CAD build for the part. Positions are in the model's coordinates, mm. A direction names the side the tool comes from. Coordinates: 2 decimals unless noted, no trailing zeros. Loops run counter-clockwise (first coordinate to the right, second up) from the corner with the lowest first, then second, coordinate; pieces in that order, holes last.
1) Wall check: line 1 along Y through (x, z) = (0, 2.9); line 2 along Y through (x, z) = (2, 2.25); line 3 along Y through (x, z) = (-23, 1.75). Give the ranges that are in metal, low to high.
2) Saw through at B-B, the plane x = 0. Give the number of separate pieces and of enclosed holes in the cut face, and give its area (3 significant figures).
3) Two-plate mould, pull along X, no slides. Class faces 4 (the flat face through (-21, -11, 6)), 5 (the flat face through (1.5, 9, 4)), 6 (the cylindrical face through (0, -22, 4)): +X half, -X half, draft (parallel to the pull), parting line (faces both ways), or undercut.
4) Pin check, flat tips, straight feed: pin 1 Ø3 at (x, y) = (14, -16.5) entering from -Z; pin 2 Ø1 at (x, y) = (-20, -15) entering from +Z; pin 3 Ø2.5 at (x, y) = (-23, 0) entering from -Z. Stop position of each tip, or through.
5) Saw through at C-C, the plane x = 8. Write the cut outline in (y, z), and give its area (3 significant figures).
6) Which spindle directions (+Z, -Z, +X, -X, +Y, -Y) get a long thin tool onto all of the face, cutting with end or side? Do faces 1 (the flat face through (20.5, 5, 4)), 2 (the flat face through (-10.5, 18, 5)), 3 (the cylindrical face through (2.93, -21.1, 4.03)). Say none if no direction does.
7) Saw through at A-A, the plane z = 7. Write the cut outline in (x, y), and give its area (3 significant figures).
```python
from build123d import *

# Parameters (mm, degrees)
F1_DEPTH         = 2
F2_W             = 5
F2_H             = 5
F3_DEPTH         = 4
F4_DEPTH         = 6
F5_R             = 1
F7_D             = 2
F7_CBORE_D       = 4.2
F7_CBORE_DEPTH   = 1.5
F2_W_2           = 15
F2_H_2           = 13
F8_DEPTH         = 25
F9_SIZE          = 1.99999
F10_R            = 1.5
F11_DEPTH        = 4
F14_DEPTH        = 6
F16_DEPTH        = 1.5
F18_DEPTH        = 1
F19_D            = 3
F20_W            = 4
F20_H            = 4
F21_DEPTH        = 4
F22_R            = 0.99999
F24_D            = 1.8
F24_DEPTH        = 5
F24_TIP          = 0.5407745571
F24_ON_F13_D     = 1.8
F24_ON_F13_DEPTH = 5
F24_ON_F13_TIP   = 0.5407745571
F24_ON_F23_D     = 1.8
F24_ON_F23_DEPTH = 5
F24_ON_F23_TIP   = 0.5407745571
F25_DEPTH        = 3
F27_DEPTH        = 2.5
F28_SIZE         = 1.99999
F29_R            = 0.99999
F30_DEPTH        = 1
F31_DEPTH        = 1
F32_DEPTH        = 1
F33_DEPTH        = 1
F34_R            = 2
F36_D            = 1.8
F36_DEPTH        = 5
F36_TIP          = 0.5407745571


# Not quite as in the source:
# - a fillet or chamfer is up to 0.001 mm smaller than in the source, because OpenCascade refuses the exact size
# - a feature names something its author has since deleted; it is built from what else it names


with BuildPart() as f1:
    # F0 (on Top) → F1 (new body)
    with BuildSketch(Plane.XY):
        with BuildLine():
            Line((-24.5, -25.5), (24.5, -25.5))
            ThreePointArc((24.5, -25.5), (25.2071067812, -25.2071067812), (25.5, -24.5))
            Line((25.5, -24.5), (25.5, 24.5))
            ThreePointArc((25.5, 24.5), (25.2071067812, 25.2071067812), (24.5, 25.5))
            Line((24.5, 25.5), (-24.5, 25.5))
            ThreePointArc((-24.5, 25.5), (-25.2071067812, 25.2071067812), (-25.5, 24.5))
            Line((-25.5, 24.5), (-25.5, -24.5))
            ThreePointArc((-25.5, -24.5), (-25.2071067812, -25.2071067812), (-24.5, -25.5))
        make_face()
    extrude(amount=F1_DEPTH)

    # F2 (on face) → F3 (join)
    with BuildSketch(Plane.XY.offset(2)):
        with Locations((-23, 0)):
            Rectangle(F2_W, F2_H)
        with Locations((0, 23)):
            Rectangle(F2_W, F2_H)
        with Locations((23, 5)):
            Rectangle(F2_W, F2_H)
        with Locations((0, -23)):
            Rectangle(F2_W, F2_H)
    extrude(amount=F3_DEPTH)

    # F2 (on face) → F4 (join)
    with BuildSketch(Plane.XY.offset(2)):
        with BuildLine():
            Line((-25.5, 24.5), (-25.5, 10.5))
            Line((-25.5, 10.5), (-10.5, 10.5))
            Line((-10.5, 10.5), (-10.5, 25.5))
            Line((-10.5, 25.5), (-24.5, 25.5))
            ThreePointArc((-24.5, 25.5), (-25.2071067812, 25.2071067812), (-25.5, 24.5))
        make_face()
    extrude(amount=F4_DEPTH)

    # F5
    f5_edges = [f1.edges().sort_by_distance(p)[0] for p in [
        (-10.5, 10.5, 5),
    ]]
    fillet(f5_edges, radius=F5_R)

    # F7 (through all)
    with Locations(Plane(origin=(0, 0, 0), x_dir=(1, 0, 0), z_dir=(0, 0, -1))):
        with Locations((-23, 0), (0, 23), (23, -5), (0, -23)):
            CounterBoreHole(F7_D / 2, F7_CBORE_D / 2, F7_CBORE_DEPTH)

    # F2 (on face) → F8 (cut)
    with BuildSketch(Plane.XY.offset(2)):
        with Locations((-3.5, -8.5)):
            Rectangle(F2_W_2, F2_H_2)
    extrude(amount=-F8_DEPTH, mode=Mode.SUBTRACT)

    # F9 (size 2 in the source; OpenCascade refuses exactly that, so slightly less here)
    f9_edges = [f1.edges().sort_by_distance(p)[0] for p in [
        (-11, -8.5, 0),
        (-3.5, -15, 0),
        (4, -8.5, 0),
        (-3.5, -2, 0),
    ]]
    chamfer(f9_edges, length=F9_SIZE)

    # F10 (on face) → F11 (join)
    with BuildSketch(Plane.XY.offset(2)):
        with BuildLine():
            Line((-24.5, -25.5), (-16.5, -25.5))
            Line((-16.5, -25.5), (-16.5, -6.5))
            Line((-16.5, -6.5), (-17.5, -5.5))
            Line((-17.5, -5.5), (-17.5, -3.5))
            ThreePointArc((-17.5, -3.5), (-17.7928932188, -2.7928932188), (-18.5, -2.5))
            Line((-18.5, -2.5), (-20.5, -2.5))
            Line((-20.5, -2.5), (-25.5, -2.5))
            Line((-25.5, -2.5), (-25.5, -24.5))
            ThreePointArc((-25.5, -24.5), (-25.2071067812, -25.2071067812), (-24.5, -25.5))
        make_face()
        with Locations((-14, -4)):
            Circle(F10_R)
    extrude(amount=F11_DEPTH)

    # F13 (on face) → F14 (cut)
    with BuildSketch(Plane.XY.offset(8)):
        Polygon((-14.5, 12.5), (-12.5, 12.5), (-12.5, 20.5), (-23.5, 20.5), (-23.5, 12.5), (-18.5, 12.5), (-18.5, 10.5), (-14.5, 10.5), align=None)
    extrude(amount=-F14_DEPTH, mode=Mode.SUBTRACT)

    # F15 (on face) → F16 (cut)
    with BuildSketch(Plane(origin=(0, 0, 0), x_dir=(1, 0, 0), z_dir=(0, 0, -1))):
        with BuildLine():
            ThreePointArc((-2.1, 23), (0, 25.1), (2.1, 23))
            Line((2.1, 23), (2.1, 25.5))
            Line((2.1, 25.5), (-2.1, 25.5))
            Line((-2.1, 25.5), (-2.1, 23))
        make_face()
        with BuildLine():
            Line((25.5, -7.1), (25.5, -2.9))
            Line((25.5, -2.9), (23, -2.9))
            ThreePointArc((23, -2.9), (24.4849242405, -3.5150757595), (25.1, -5))
            ThreePointArc((25.1, -5), (24.4849242405, -6.4849242405), (23, -7.1))
            Line((23, -7.1), (25.5, -7.1))
        make_face()
        with BuildLine():
            Line((-23, 2.1), (-25.5, 2.1))
            Line((-25.5, 2.1), (-25.5, -2.1))
            Line((-25.5, -2.1), (-23, -2.1))
            ThreePointArc((-23, -2.1), (-25.1, 0), (-23, 2.1))
        make_face()
        with BuildLine():
            Line((-2.1, -25.5), (2.1, -25.5))
            Line((2.1, -25.5), (2.1, -23))
            ThreePointArc((2.1, -23), (0, -25.1), (-2.1, -23))
            Line((-2.1, -23), (-2.1, -25.5))
        make_face()
    extrude(amount=-F16_DEPTH, mode=Mode.SUBTRACT)

    # F17 (on face) → F18 (cut)
    with BuildSketch(Plane(origin=(0, 0, 0), x_dir=(1, 0, 0), z_dir=(0, 0, -1))):
        Polygon((17.25, 18.0877132403), (14.5, 19.6754264805), (11.75, 18.0877132403), (11.75, 14.9122867597), (14.5, 13.3245735195), (17.25, 14.9122867597), align=None)
        Polygon((17.25, -0.0877132403), (17.25, 3.0877132403), (14.5, 4.6754264805), (11.75, 3.0877132403), (11.75, -0.0877132403), (14.5, -1.6754264805), align=None)
    extrude(amount=-F18_DEPTH, mode=Mode.SUBTRACT)

    # F19 (through all)
    with Locations(Plane(origin=(0, 0, 0), x_dir=(1, 0, 0), z_dir=(0, 0, -1))):
        with Locations((14.5, 16.5), (14.5, 1.5)):
            Hole(F19_D / 2)

    # F20 (on face) → F21 (join)
    with BuildSketch(Plane.XY.offset(2)):
        with Locations((23.5, 9.5)):
            Rectangle(F20_W, F20_H)
        with Locations((3.5, 9.5)):
            Rectangle(F20_W, F20_H)
        with BuildLine():
            Line((2.5, 20.5), (25.5, 20.5))
            Line((25.5, 20.5), (25.5, 24.5))
            ThreePointArc((25.5, 24.5), (25.2071067812, 25.2071067812), (24.5, 25.5))
            Line((24.5, 25.5), (2.5, 25.5))
            Line((2.5, 25.5), (2.5, 20.5))
        make_face()
        with BuildLine():
            Line((25.5, -24.5), (25.5, -20.5))
            Line((25.5, -20.5), (20.5, -20.5))
            Line((20.5, -20.5), (20.5, -25.5))
            Line((20.5, -25.5), (24.5, -25.5))
            ThreePointArc((24.5, -25.5), (25.2071067812, -25.2071067812), (25.5, -24.5))
        make_face()
    extrude(amount=F21_DEPTH)

    # F22 (radius 1 in the source; OpenCascade refuses exactly that, so slightly less here)
    f22_edges = [f1.edges().sort_by_distance(p)[0] for p in [
        (5.5, 7.5, 4),
        (1.5, 7.5, 4),
        (1.5, 11.5, 4),
        (20.5, 7.5, 4),
        (5.5, 11.5, 4),
        (21.5, 11.5, 4),
    ]]
    fillet(f22_edges, radius=F22_R)

    # F24
    with Locations(Plane.XY.offset(6)):
        with Locations((-22, -22), (-22, -7)):
            Hole(F24_D / 2, depth=F24_DEPTH)
            with Locations((0, 0, -(F24_DEPTH + F24_TIP / 2))):  # 118° drill point
                Cone(0, F24_D / 2, F24_TIP, mode=Mode.SUBTRACT)

    # F24 on F13
    with Locations(Plane.XY.offset(8)):
        with Locations((-22.5, 22.5), (-13.5, 22.5)):
            Hole(F24_ON_F13_D / 2, depth=F24_ON_F13_DEPTH)
            with Locations((0, 0, -(F24_ON_F13_DEPTH + F24_ON_F13_TIP / 2))):  # 118° drill point
                Cone(0, F24_ON_F13_D / 2, F24_ON_F13_TIP, mode=Mode.SUBTRACT)

    # F24 on F23
    with Locations(Plane.XY.offset(6)):
        with Locations((3.5, 9.5), (23.5, 9.5)):
            Hole(F24_ON_F23_D / 2, depth=F24_ON_F23_DEPTH)
            with Locations((0, 0, -(F24_ON_F23_DEPTH + F24_ON_F23_TIP / 2))):  # 118° drill point
                Cone(0, F24_ON_F23_D / 2, F24_ON_F23_TIP, mode=Mode.SUBTRACT)

    # F25 (add): a face of the model
    f25_faces = [f1.faces().sort_by_distance(p)[0] for p in [
        (-23.5, 16.5, 5),
    ]]
    extrude(f25_faces, amount=F25_DEPTH)

    # F26 (on face) → F27 (cut)
    with BuildSketch(Plane(origin=(0, 0, 0), x_dir=(1, 0, 0), z_dir=(0, 0, -1))):
        with BuildLine():
            Line((-20.5, -21.5), (-21.5, -21.5))
            Line((-21.5, -21.5), (-25.5, -21.5))
            Line((-25.5, -21.5), (-25.5, -24.5))
            ThreePointArc((-25.5, -24.5), (-25.2071067812, -25.2071067812), (-24.5, -25.5))
            Line((-24.5, -25.5), (-21.5, -25.5))
            Line((-21.5, -25.5), (-21.5, -24.5))
            Line((-21.5, -24.5), (-15, -24.5))
            Line((-15, -24.5), (-15, -21))
            Line((-15, -21), (-15, -18.5))
            Line((-15, -18.5), (-20.5, -18.5))
            Line((-20.5, -18.5), (-20.5, -21.5))
        make_face()
    extrude(amount=-F27_DEPTH, mode=Mode.SUBTRACT)

    # F28 (size 2 in the source; OpenCascade refuses exactly that, so slightly less here)
    f28_edges = [f1.edges().sort_by_distance(p)[0] for p in [
        (-17.75, 18.5, 2),
    ]]
    chamfer(f28_edges, length=F28_SIZE)

    # F29 (radius 1 in the source; OpenCascade refuses exactly that, so slightly less here)
    f29_edges = [f1.edges().sort_by_distance(p)[0] for p in [
        (-25.5, 21.5, 1.25),
        (-21.5, 24.5, 1.25),
        (-15, 24.5, 1.25),
    ]]
    fillet(f29_edges, radius=F29_R)

    # F30 (add): faces of the model
    f30_faces = [f1.faces().sort_by_distance(p)[0] for p in [
        (-2.5, 23, 4),
        (-2.5, -23, 4),
        (20.5, -23, 4),
    ]]
    extrude(f30_faces, amount=F30_DEPTH)

    # F31 (add): a face of the model
    f31_faces = [f1.faces().sort_by_distance(p)[0] for p in [
        (2.5, -23, 4),
    ]]
    extrude(f31_faces, amount=F31_DEPTH)

    # F32 (add): a face of the model
    f32_faces = [f1.faces().sort_by_distance(p)[0] for p in [
        (23, 2.5, 4),
    ]]
    extrude(f32_faces, amount=F32_DEPTH)

    # F33 (add): a face of the model
    f33_faces = [f1.faces().sort_by_distance(p)[0] for p in [
        (-23, 2.5, 4),
    ]]
    extrude(f33_faces, amount=F33_DEPTH)

    # F34
    f34_edges = [f1.edges().sort_by_distance(p)[0] for p in [
        (19.5, -20.5, 4),
        (20.5, 1.5, 4),
        (3.5, -20.5, 4),
        (-3.5, -20.5, 4),
        (-3.5, 20.5, 4),
        (-20.5, 3.5, 4),
    ]]
    fillet(f34_edges, radius=F34_R)

    # F36
    with Locations(Plane(origin=(0, 0, 0), x_dir=(1, 0, 0), z_dir=(0, 0, -1))):
        with Locations((-23, -18.5), (-23, 18.5), (23, -23), (23, 23)):
            Hole(F36_D / 2, depth=F36_DEPTH)
            with Locations((0, 0, -(F36_DEPTH + F36_TIP / 2))):  # 118° drill point
                Cone(0, F36_D / 2, F36_TIP, mode=Mode.SUBTRACT)


solid = f1.part
```
Data:
1. line 1: y = -25.5 to -24, -22 to -20.5, 20.5 to 22, 24 to 25.5
1. line 2: y = -25.5 to -20.56, 7.63 to 11.37, 20.5 to 25.5
1. line 3: y = -25.5 to -19.4, -17.6 to -1, 1 to 17.6, 19.4 to 21.5
2. separate pieces: 4
2. enclosed holes: 0
2. area: 80.2 mm2
3. face 4: draft
3. face 5: -X half
3. face 6: undercut
4. pin 1: stops at z = 1
4. pin 2: stops at z = 6
4. pin 3: stops at z = 1.5
5. outline: (-25.5, 0) - (25.5, 0) - (25.5, 6) - (20.5, 6) - (20.5, 2) - (-25.5, 2) - close
5. area: 122 mm2
6. face 1: +Z, -X
6. face 2: +Z, +Y, -Y
6. face 3: +Z
7. outline: (-25.5, 10.5) - (-18.5, 10.5) - (-18.5, 12.5) - (-20.5, 12.5) - (-20.5, 20.5) - (-12.5, 20.5) - (-12.5, 12.5) - (-14.5, 12.5) - (-14.5, 10.5) - (-11.5, 10.5) arc R1 ccw to (-10.5, 11.5) - (-10.5, 25.5) - (-24.5, 25.5) arc R1 ccw to (-25.5, 24.5) - close; hole circle Ø1.8 at (-22.5, 22.5); hole circle Ø1.8 at (-13.5, 22.5)
7. area: 147 mm2
